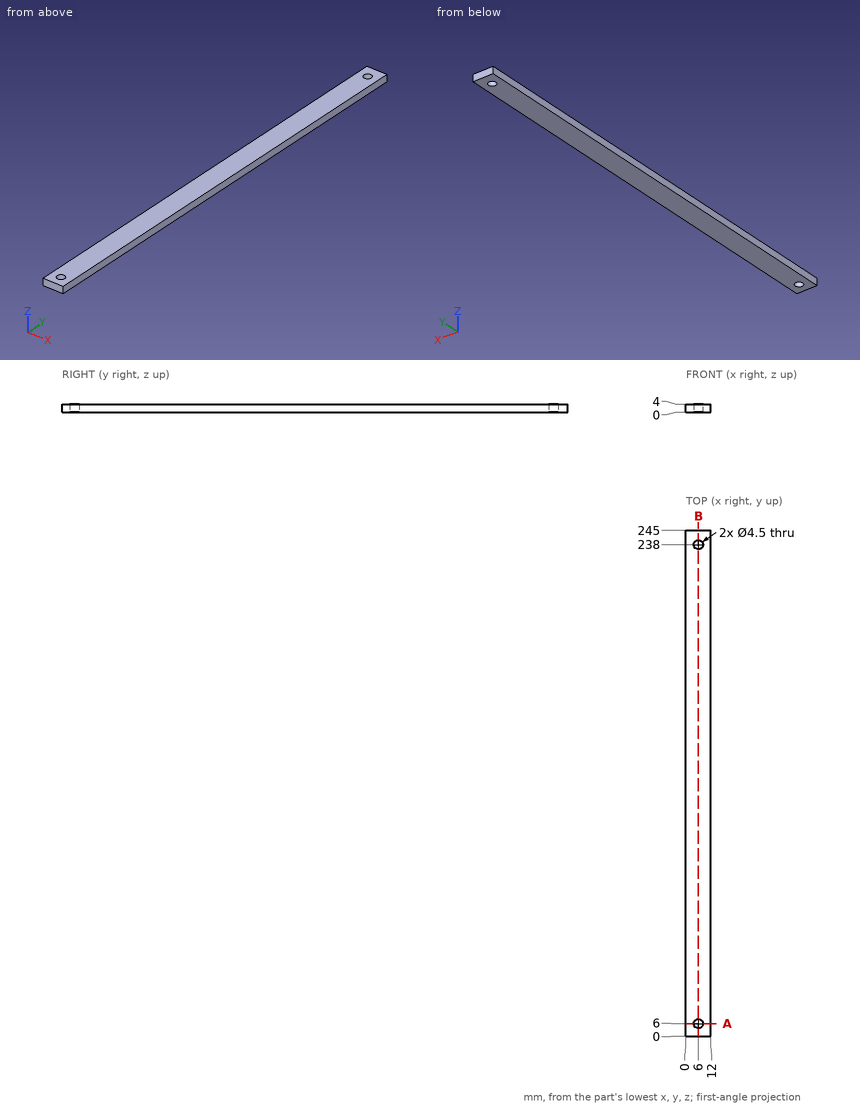
Job drawing, mm, ordinate dimensions from the low corner. One solid piece. Coordinates: 2 decimals unless noted, no trailing zeros. Order: outer loops, then holes, each group sorted by start corner. A loop starts at its lowest first (then second) coordinate and runs counter-clockwise, first axis right, second up. Notation, with made-up numbers: (-9, -18) - (25, -18) arc R31 cw to (25, 9) - close; hole circle Ø8 at (49, 39.5). An arc over 180 degrees is marked (long way). Use CSV: the item, a comma, the result in double quotes.
Item 1: Saw through at A-A on y = 6. Give the cut face in (x, z), and give its area (3 significant figures).
Solved:
outline,"(0, 0) - (3.75, 0) - (3.75, 4) - (0, 4) - close; (8.25, 0) - (12, 0) - (12, 4) - (8.25, 4) - close"
area,"30.0 mm²"
Item 2: Saw through at B-B on x = 6. Give the cut face in (y, z), and give its area (3 significant figures).
Solved:
outline,"(0, 0) - (3.75, 0) - (3.75, 4) - (0, 4) - close; (8.25, 0) - (235.75, 0) - (235.75, 4) - (8.25, 4) - close; (240.25, 0) - (245, 0) - (245, 4) - (240.25, 4) - close"
area,"944 mm²"
Item 3: Probe probe 1 along Y at (x, z) = (6, 2.05); probe 2 along X at (y, z) = (238, 2.3); probe 3 along Y at (x, z) = (7.5, 0.5). List the from-to ranges inside material, lowest first.
Solved:
probe 1,"y = 0 to 3.75, 8.25 to 235.75, 240.25 to 245"
probe 2,"x = 0 to 3.75, 8.25 to 12"
probe 3,"y = 0 to 4.32, 7.68 to 236.32, 239.68 to 245"
